Verification items for the finished model (mm, model axes). A direction names the side the tool comes from. Coordinates: 2 decimals unless noted, no trailing zeros. Loops run counter-clockwise (first coordinate to the right, second up) from the corner with the lowest first, then second, coordinate; pieces in that order, holes last. Notation, with made-up numbers: (60.5, 27) - (69.5, 27) arc R26 ccw to (69.5, 51) - close; hole circle Ø9 at (24.25, -31). An arc over 180 degrees is marked (long way). One line per item, written item: value. Start each with the question number.
(1) Section check B-B (y = -1.75). Count the separate pieces of the cut face and the enclosed holes in it, plus the area to 3 significant figures.
(2) Gauge pin test, flat ends, axial feed: P1, Ø3, axis at y = 2.5, z = 21, coming from the -X side; P2, Ø1, axis at y = -3, z = -37, coming from the +X side; P3, Ø2, axis at y = 3, z = -21.5, coming from the -X side. Record the tip position at first contact, or that the pin passes through.
(3) Set-up check for faces 1 (the face through (-4.31, 2.535, 5.67)), 2 (the face through (-4.35, -2.465, 5.67)), 3 (the face through (0, 5, 96)): record each of +Z, -Z, +X, -X, +Y, -Y from which the full face is reachable in a straight line by a thin tool's end or side.
(4) Thickness scan on probe 1 along X at (y, z) = (0, 82.5); probe 2 along Z at (x, y) = (0, 1.7); probe 3 along X at (y, z) = (-3.25, 90). Record the ranges inside material, lowest first. Write a range as [from, to].
(5) Section check A-A (z = 55). Record the boundary of the cut face in (x, y), plus the area to 3 significant figures.
```python
from build123d import *

# Parameters (mm, degrees)
BOSS_EXTRUDE1_DEPTH     = 100
CUT_EXTRUDE1_DEPTH      = 6
CUT_EXTRUDE1_DEPTH_BACK = 6
SKETCH5_R               = 3
CUT_EXTRUDE2_DEPTH      = 6.0000001
CUT_EXTRUDE2_DEPTH_BACK = 6.0000001


with BuildPart() as part:
    # Sketch1 → Boss-Extrude1 (new body, symmetric)
    with BuildSketch(Plane.XY):
        Polygon((-5.773502692, 0), (-2.886751346, -5), (2.886751346, -5), (5.773502692, 0), (2.886751346, 5), (-2.886751346, 5), align=None)
    extrude(amount=BOSS_EXTRUDE1_DEPTH, both=True)

    # Sketch2 → Cut-Extrude1 (cut, two sides)
    with BuildSketch(Plane(origin=(0, 0, 0), x_dir=(1, 0, 0), z_dir=(0, 1, 0))) as cut_extrude1_sk:
        Polygon((5.773502692, 100), (-5.773502692, 88.452994616), (-5.773502692, 100), align=None)
    extrude(amount=CUT_EXTRUDE1_DEPTH, mode=Mode.SUBTRACT)
    extrude(cut_extrude1_sk.sketch, amount=-CUT_EXTRUDE1_DEPTH_BACK, mode=Mode.SUBTRACT)

    # Sketch4 → section 0 of loft1
    with BuildSketch(Plane.ZY.offset(155), mode=Mode.PRIVATE) as loft1_s0:
        Polygon((-97.113248654, 5), (-100, 0), (-97.113248654, -5), (-91.339745962, -5), (-88.452994616, 0), (-91.339745962, 5), align=None)
    # loft up to a face of the part (loft1)
    loft([loft1_s0.sketch, part.faces().sort_by_distance((0, 0, -94.226497308))[0]])

    # Sketch5 → Cut-Extrude2 (cut, two sides)
    with BuildSketch(Plane(origin=(0, 0, 0), x_dir=(1, 0, 0), z_dir=(0, 1, 0))) as cut_extrude2_sk:
        with Locations((0, -90)):
            Circle(SKETCH5_R)
        with Locations((-145, 94.226497308)):
            Circle(SKETCH5_R)
    extrude(amount=CUT_EXTRUDE2_DEPTH, mode=Mode.SUBTRACT)
    extrude(cut_extrude2_sk.sketch, amount=-CUT_EXTRUDE2_DEPTH_BACK, mode=Mode.SUBTRACT)


solid = part.part
```
Responses:
1. separate pieces: 1
1. enclosed holes: 2
1. area: 3,270 mm²
2. P1: stops at x = -5.2
2. P2: stops at x = 4.33
2. P3: stops at x = -4.62
3. face 1: +Z, -X, +Y
3. face 2: +Z, -X, -Y
3. face 3: +Z, -Z, +X, -X, +Y
4. probe 1: x = [-5.77, 5.77]
4. probe 2: z = [-99.02, 87], [93, 100]
4. probe 3: x = [-3.9, -3], [3, 3.9]
5. outline: (-5.77, 0) - (-2.89, -5) - (2.89, -5) - (5.77, 0) - (2.89, 5) - (-2.89, 5) - close
5. area: 86.6 mm²
